from build123d import *

# Parameters (mm, degrees)
TUBE001_R               = 10
TUBE001_R_2             = 6
TUBE001_DEPTH           = 14
SKETCH083_R             = 8
PAD059_DEPTH            = 50.5
SKETCH277_R             = 2.25
PAD114_DEPTH            = 5
SKETCH284_R             = 2.25
PAD119_DEPTH            = 21
BODY035_PLACEMENT_ANGLE = 180


with BuildPart() as tube001:
    # Tube001 → Tube001 (new body)
    with BuildSketch(Plane(origin=(-76, 7, 1), x_dir=(1, 0, 0), z_dir=(0, -1, 0))):
        Circle(TUBE001_R)
        Circle(TUBE001_R_2, mode=Mode.SUBTRACT)
    extrude(amount=TUBE001_DEPTH)


with BuildPart() as cut:
    # Sketch083 → Pad059 (new body)
    with BuildSketch(Plane.XZ):
        Circle(SKETCH083_R)
    extrude(amount=-PAD059_DEPTH)

    # Sketch277 (on Face2 of Pad059) → Pad114 (join)
    with BuildSketch(Plane.XZ):
        Circle(SKETCH277_R)
    extrude(amount=PAD114_DEPTH)

    # Sketch284 (on Face3 of Pad114) → Pad119 (join)
    with BuildSketch(Plane(origin=(0, 50.5, 0), x_dir=(1, 0, 0), z_dir=(0, 1, 0))):
        Circle(SKETCH284_R)
    extrude(amount=PAD119_DEPTH)


with BuildPart() as cut_1:
    # Body035 placement: moved
    add(cut.part.moved(Location((-76, 30, 1))).rotate(Axis((-76, 30, 1), (1, 0, 0)), BODY035_PLACEMENT_ANGLE))

    # Cut: cut Tube001
    add(tube001.part, mode=Mode.SUBTRACT)


solid = cut_1.part
Source: CAD feature listing. Evaluate the final solid. Frame: model axes, mm. A direction names the side the tool comes from. Round coordinates to 2 decimals unless told otherwise and drop trailing zeros. Loops run counter-clockwise (first coordinate to the right, second up) from the corner with the lowest first, then second, coordinate; pieces in that order, holes last. Notation, with made-up numbers: M 61.25,-9.75 L 99.25,-9.75 A24 ccw 99.25,4.25 Z; hole C 29.5,10.5 d5. An arc over 180 degrees is marked long. Answer as CSV lines item,"result".
Q1. Cut plane D-D (x = -72.25). Return the cut outline in (y, z), plus the area to 3 significant figures.
Verdict:
outline,"M -20.5,-6.07 L -7,-6.07 L -7,-3.68 L 7,-3.68 L 7,-6.07 L 30,-6.07 L 30,8.07 L 7,8.07 L 7,5.68 L -7,5.68 L -7,8.07 L -20.5,8.07 Z"
area,"647 mm^2"
Q2. Cut plane A-A (x = -76). Return the cut outline in (y, z).
Verdict:
outline,"M -41.5,-1.25 L -20.5,-1.25 L -20.5,-7 L -7,-7 L -7,-5 L 7,-5 L 7,-7 L 30,-7 L 30,-1.25 L 35,-1.25 L 35,3.25 L 30,3.25 L 30,9 L 7,9 L 7,7 L -7,7 L -7,9 L -20.5,9 L -20.5,3.25 L -41.5,3.25 Z"
Q3. Pull-direction query (Y, two-part tool) for faces 1 (the face through (-82.349, 18.661, 5.868)), 2 (the face through (-76, -41.5, 1)), 3 (the face through (-78, -7, 7)), 4 (the face through (-78, 7, 7)); classes: +Y half, -Y half, draft (parallel to the pull), parting line (faces both ways), or undercut.
Verdict:
face 1,"draft"
face 2,"-Y half"
face 3,"undercut"
face 4,"undercut"
Q4. Line query: line 1 along Y through (x, z) = (-79.75, -5.75); line 2 along Y through (x, z) = (-76.5, -4.75); line 3 along Z through (x, y) = (-76.5, 21.5). Output: solid intervals per line, ascending.
Verdict:
line 1,"y = -20.5 to -7, 7 to 30"
line 2,"y = -20.5 to 30"
line 3,"z = -6.98 to 8.98"
Q5. Cut plane C-C (y = -26). Return the cut outline in (x, z), plus the area to 3 significant figures.
Verdict:
outline,"C -76,1 d4.5"
area,"15.9 mm^2"
Q6. Reachability of faces 5 (the face through (-82, 0, 1)), 6 (the face through (-74, 30, 3)), 7 (the face through (-73.92, -30.85, 0.14)) from +Z, -Z, +X, -X, +Y, -Y: full face, straight path, thin tool, end or side. Return the list, or none.
Verdict:
face 5,"none"
face 6,"+Y"
face 7,"-Y"
Q7. Cut plane B-B (z = 1). Return the cut outline in (x, y), plus the area to 3 significant figures.
Verdict:
outline,"M -84,-20.5 L -78.25,-20.5 L -78.25,-41.5 L -73.75,-41.5 L -73.75,-20.5 L -68,-20.5 L -68,-7 L -70,-7 L -70,7 L -68,7 L -68,30 L -73.75,30 L -73.75,35 L -78.25,35 L -78.25,30 L -84,30 L -84,7 L -82,7 L -82,-7 L -84,-7 Z"
area,"869 mm^2"
Q8. Contact query for flat-ended pins moving along their axis: pin 1 (3 mm diameter, centred on y = -23, z = 0.5, fed in from +X); pin 2 (2 mm diameter, centred on x = -79.5, z = -4.5, fed in from -Y); pin 3 (8 mm diameter, centred on x = -80, y = -19, fed in from -Z); pin 4 (4 mm diameter, centred on x = -79.5, z = -2.5, fed in from +Y). Output: stop coordinate, or through.
Verdict:
pin 1,"stops at x = -73.75"
pin 2,"stops at y = -20.5"
pin 3,"stops at z = -7"
pin 4,"stops at y = 30"
